Here's how the part is built. I have some questions about the finished solid (model axes, mm). Face numbers are marked on the shaded views. A direction names the side the tool comes from. Coordinates: 2 decimals unless noted, no trailing zeros. Write each loop counter-clockwise with the first axis right and the second up, starting at its lowest first coordinate (ties: lowest second). Pieces come first, ordered by that corner, then holes. Notation, with made-up numbers: M 26.25,-9 L 62.25,-9 A26 ccw 62.25,28 Z; hole C 87,-39.75 d11. An arc over 180 degrees is marked long. Use one line per item in the form item = value. Start each with the question number.
1. I want a section at A-A, the plane x = -18.5. List the corners of the cut face in (y, z) for me.
2. I want a section at D-D, the plane z = 45.5. List the corners of the cut face in (x, y) for me.
3. I want a section at C-C, the plane z = 55. List the corners of the cut face in (x, y) for me, plus the area to 3 significant figures.
4. Thinking about a two-plate mould opening in Z: for the marked faces 5, 6 and 7, which applies, released by +Z, released by -Z, zero draft, split by the parting line, or undercut?
5. I want a section at B-B, the plane z = 12. List the corners of the cut face in (x, y) for me.
6. I'm going to push flat-ended pins straight in: pin 1 Ø4.5 at (x, z) = (30.5, 56.5) entering from -Y; pin 2 Ø5 at (x, y) = (30, -9.5) entering from +Z; pin 3 Ø1 at (x, y) = (21, -24) entering from +Z. Where does each tip first touch, or does it pass through?
7. On a 3-axis mill with a long thin cutter (end or side, diameter ignored), from which of +Z, -Z, +X, -X, +Y, -Y can I reach the whole of each face in a straight line? I mean the marked faces 1, 2, 3 and 4. Say none if no direction works.
8. Please list where these lines run through material, in increasing order: line 1 along Z through (x, y) = (-32, -13); line 2 along X through (y, z) = (-7, 3); line 3 along X through (y, z) = (-4, 9). Write a range as [from, to].
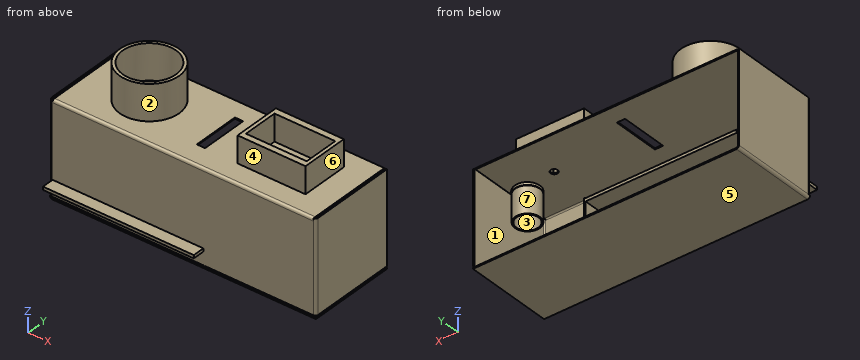
from build123d import *

# Parameters (mm, degrees)
SKETCH1_W                    = 150
SKETCH1_H                    = 50
BASE_FLANGE1_DEPTH           = 0.7366
EDGE_FLANGE2_STRIP_W         = 4.4196
EDGE_FLANGE2_STRIP_H         = 0.7366
EDGE_FLANGE2_STRIP_CUT_DEPTH = 50
EDGE_FLANGE2_DEPTH           = 50
EDGE_FLANGE3_STRIP_W         = 4.4196
EDGE_FLANGE3_STRIP_H         = 0.7366
EDGE_FLANGE3_STRIP_CUT_DEPTH = 51.7366
EDGE_FLANGE3_DEPTH           = 51.7366
EDGE_FLANGE5_STRIP_W         = 4.4196
EDGE_FLANGE5_STRIP_H         = 0.7366
EDGE_FLANGE5_STRIP_CUT_DEPTH = 51.7366
EDGE_FLANGE5_DEPTH           = 51.7366
EDGE_FLANGE6_STRIP_W         = 4.4196
EDGE_FLANGE6_STRIP_H         = 0.7366
EDGE_FLANGE6_STRIP_CUT_DEPTH = 147.0536
EDGE_FLANGE6_DEPTH           = 147.0536
SKETCH38_W                   = 4.66509895
SKETCH38_H                   = 26.811141958
CUT_EXTRUDE1_DEPTH           = 2
SKETCH40_R                   = 16.736303479
SKETCH40_R_2                 = 14.955594907
BOSS_EXTRUDE4_DEPTH          = 20
SKETCH42_W                   = 0.865074657
SKETCH42_H                   = 50
BOSS_EXTRUDE5_DEPTH          = 10
SKETCH57_W                   = 1.770321067
SKETCH57_H                   = 56.722896859
BOSS_EXTRUDE7_DEPTH          = 85
SKETCH60_W                   = 38.271407539
SKETCH60_H                   = 26.924897386
SKETCH60_W_2                 = 34.235775553
SKETCH60_H_2                 = 20.047107357
BOSS_EXTRUDE8_DEPTH          = 15
SKETCH61_R                   = 2.019782533
CUT_EXTRUDE3_DEPTH           = 2
SKETCH62_R                   = 1.571954748
BOSS_EXTRUDE9_DEPTH          = 3
SKETCH63_R                   = 7.10603058
BOSS_EXTRUDE10_DEPTH         = 1.5
SKETCH64_R                   = 6.980489156
SKETCH64_R_2                 = 6.226740222
BOSS_EXTRUDE11_DEPTH         = 15


# Sheet-metal steps are written as plain solids
with BuildPart() as part:
    # Sketch1 → Base-Flange1 (new body)
    with BuildSketch(Plane.XY):
        Rectangle(SKETCH1_W, SKETCH1_H)
    extrude(amount=-BASE_FLANGE1_DEPTH)

    # Edge-Flange2 strip (across the edge) → Edge-Flange2 strip cut (cut)
    with BuildSketch(Plane(origin=(-75, 25, 0), x_dir=(1, 0, 0), z_dir=(0, -1, 0))):
        with Locations((-0.7366, -0.3683)):
            Rectangle(EDGE_FLANGE2_STRIP_W, EDGE_FLANGE2_STRIP_H)
    extrude(amount=EDGE_FLANGE2_STRIP_CUT_DEPTH, mode=Mode.SUBTRACT)

    # Edge-Flange2 section (across the edge) → Edge-Flange2 (add)
    with BuildSketch(Plane(origin=(-75, 25, 0), x_dir=(1, 0, 0), z_dir=(0, -1, 0))):
        with BuildLine():
            Line((0, 0.7366), (0, 52.4732))
            Line((0, 52.4732), (0.7366, 52.4732))
            Line((0.7366, 52.4732), (0.7366, 0.7366))
            ThreePointArc((0.7366, 0.7366), (0.952345145, 0.215745145), (1.4732, 0))
            Line((1.4732, 0), (1.4732, -0.7366))
            ThreePointArc((1.4732, -0.7366), (0.43149029, -0.30510971), (0, 0.7366))
        make_face()
    extrude(amount=EDGE_FLANGE2_DEPTH)

    # Edge-Flange3 strip (across the edge) → Edge-Flange3 strip cut (cut)
    with BuildSketch(Plane(origin=(-74.2634, -25, 52.4732), x_dir=(0, 1, 0), z_dir=(0, 0, -1))):
        with Locations((-0.7366, -0.3683)):
            Rectangle(EDGE_FLANGE3_STRIP_W, EDGE_FLANGE3_STRIP_H)
    extrude(amount=EDGE_FLANGE3_STRIP_CUT_DEPTH, mode=Mode.SUBTRACT)

    # Edge-Flange3 section (across the edge) → Edge-Flange3 (add)
    with BuildSketch(Plane(origin=(-74.2634, -25, 52.4732), x_dir=(0, 1, 0), z_dir=(0, 0, -1))):
        with BuildLine():
            Line((0, 0.7366), (0, 149.2634))
            Line((0, 149.2634), (0.7366, 149.2634))
            Line((0.7366, 149.2634), (0.7366, 0.7366))
            ThreePointArc((0.7366, 0.7366), (0.952345145, 0.215745145), (1.4732, 0))
            Line((1.4732, 0), (1.4732, -0.7366))
            ThreePointArc((1.4732, -0.7366), (0.43149029, -0.30510971), (0, 0.7366))
        make_face()
    extrude(amount=EDGE_FLANGE3_DEPTH)

    # Edge-Flange5 strip (across the edge) → Edge-Flange5 strip cut (cut)
    with BuildSketch(Plane(origin=(75, -24.2634, 52.4732), x_dir=(-1, 0, 0), z_dir=(0, 0, -1))):
        with Locations((-0.7366, -0.3683)):
            Rectangle(EDGE_FLANGE5_STRIP_W, EDGE_FLANGE5_STRIP_H)
    extrude(amount=EDGE_FLANGE5_STRIP_CUT_DEPTH, mode=Mode.SUBTRACT)

    # Edge-Flange5 section (across the edge) → Edge-Flange5 (add)
    with BuildSketch(Plane(origin=(75, -24.2634, 52.4732), x_dir=(-1, 0, 0), z_dir=(0, 0, -1))):
        with BuildLine():
            Line((0, 0.7366), (0, 49.2634))
            Line((0, 49.2634), (0.7366, 49.2634))
            Line((0.7366, 49.2634), (0.7366, 0.7366))
            ThreePointArc((0.7366, 0.7366), (0.952345145, 0.215745145), (1.4732, 0))
            Line((1.4732, 0), (1.4732, -0.7366))
            ThreePointArc((1.4732, -0.7366), (0.43149029, -0.30510971), (0, 0.7366))
        make_face()
    extrude(amount=EDGE_FLANGE5_DEPTH)

    # Edge-Flange6 strip (across the edge) → Edge-Flange6 strip cut (cut)
    with BuildSketch(Plane(origin=(-73.5268, -24.2634, 52.4732), x_dir=(0, 0, -1), z_dir=(1, 0, 0))):
        with Locations((-0.7366, -0.3683)):
            Rectangle(EDGE_FLANGE6_STRIP_W, EDGE_FLANGE6_STRIP_H)
    extrude(amount=EDGE_FLANGE6_STRIP_CUT_DEPTH, mode=Mode.SUBTRACT)

    # Edge-Flange6 section (across the edge) → Edge-Flange6 (add)
    with BuildSketch(Plane(origin=(-73.5268, -24.2634, 52.4732), x_dir=(0, 0, -1), z_dir=(1, 0, 0))):
        with BuildLine():
            Line((0, 0.7366), (0, 49.2634))
            Line((0, 49.2634), (0.7366, 49.2634))
            Line((0.7366, 49.2634), (0.7366, 0.7366))
            ThreePointArc((0.7366, 0.7366), (0.952345145, 0.215745145), (1.4732, 0))
            Line((1.4732, 0), (1.4732, -0.7366))
            ThreePointArc((1.4732, -0.7366), (0.43149029, -0.30510971), (0, 0.7366))
        make_face()
    extrude(amount=EDGE_FLANGE6_DEPTH)

    # Sketch38 → Cut-Extrude1 (cut)
    with BuildSketch(Plane.XY.offset(52.4732)):
        with Locations((0, 1.125354672)):
            Rectangle(SKETCH38_W, SKETCH38_H)
    extrude(amount=-CUT_EXTRUDE1_DEPTH, mode=Mode.SUBTRACT)

    # Sketch40 → Boss-Extrude4 (add)
    with BuildSketch(Plane.XY.offset(52.4732)):
        with Locations((-40.204479975, 1.659887055)):
            Circle(SKETCH40_R)
        with Locations((-40.204479975, 1.659887055)):
            Circle(SKETCH40_R_2, mode=Mode.SUBTRACT)
    extrude(amount=BOSS_EXTRUDE4_DEPTH)

    # Sketch42 → Boss-Extrude5 (add)
    with BuildSketch(Plane.XY):
        with Locations((11.975597677, 0)):
            Rectangle(SKETCH42_W, SKETCH42_H)
    extrude(amount=BOSS_EXTRUDE5_DEPTH)

    # Sketch57 → Boss-Extrude7 (add)
    with BuildSketch(Plane.ZY.offset(-11.543060348)):
        with Locations((8.882085538, -3.36144843)):
            Rectangle(SKETCH57_W, SKETCH57_H)
    extrude(amount=BOSS_EXTRUDE7_DEPTH)

    # Sketch60 → Boss-Extrude8 (add)
    with BuildSketch(Plane.XY.offset(52.4732)):
        with Locations((40.051357612, 0.865314599)):
            Rectangle(SKETCH60_W, SKETCH60_H)
        with Locations((40.096607613, 0.750841138)):
            Rectangle(SKETCH60_W_2, SKETCH60_H_2, mode=Mode.SUBTRACT)
    extrude(amount=BOSS_EXTRUDE8_DEPTH)

    # Sketch61 → Cut-Extrude3 (cut)
    with BuildSketch(Plane(origin=(0, 0, 51.7366), x_dir=(-1, 0, 0), z_dir=(0, 0, -1))):
        with Locations((-47.658560575, 2.019782533)):
            Circle(SKETCH61_R)
    extrude(amount=-CUT_EXTRUDE3_DEPTH, mode=Mode.SUBTRACT)

    # Sketch62 → Boss-Extrude9 (add)
    with BuildSketch(Plane(origin=(0, 0, 51.7366), x_dir=(-1, 0, 0), z_dir=(0, 0, -1))):
        with Locations(Location((-63.948086172, 1.147200329, 0), (0, 0, 180))):
            Circle(SKETCH62_R)
    extrude(amount=BOSS_EXTRUDE9_DEPTH)

    # Sketch63 → Boss-Extrude10 (add)
    with BuildSketch(Plane(origin=(0, 0, 48.7366), x_dir=(-1, 0, 0), z_dir=(0, 0, -1))):
        with Locations((-63.631248371, 0.988840217)):
            Circle(SKETCH63_R)
    extrude(amount=BOSS_EXTRUDE10_DEPTH)

    # Sketch64 → Boss-Extrude11 (add)
    with BuildSketch(Plane(origin=(0, 0, 47.2366), x_dir=(-1, 0, 0), z_dir=(0, 0, -1))):
        with Locations(Location((-63.746933468, 0.733116553, 0), (0, 0, 181.202812621))):
            Circle(SKETCH64_R)
        with Locations((-63.746933468, 0.733116553)):
            Circle(SKETCH64_R_2, mode=Mode.SUBTRACT)
    extrude(amount=BOSS_EXTRUDE11_DEPTH)


solid = part.part
Answer list:
q1.outline = M -31.72,8 L -25,8 L -25,0.74 L -24.26,0.74 L -24.26,8 L 25,8 L 25,9.77 L -24.26,9.77 L -24.26,51 A0.74 cw -23.53,51.74 L 25,51.74 L 25,52.47 L -23.53,52.47 A1.47 ccw -25,51 L -25,9.77 L -31.72,9.77 Z; M -25,-0.74 L 25,-0.74 L 25,0 L -25,0 Z
q2.outline = M -75,-23.53 A1.47 ccw -73.53,-25 L 73.53,-25 A1.47 ccw 75,-23.53 L 75,25 L 74.26,25 L 74.26,-23.53 A0.74 cw 73.53,-24.26 L -73.53,-24.26 A0.74 cw -74.26,-23.53 L -74.26,25 L -75,25 Z; C 63.75,0.73 d13.96; hole C 63.75,0.73 d12.45
q3.outline = C -40.2,1.66 d33.47; M 20.92,-12.6 L 59.19,-12.6 L 59.19,14.33 L 20.92,14.33 Z; hole C -40.2,1.66 d29.91; hole M 22.98,-9.27 L 57.21,-9.27 L 57.21,10.77 L 22.98,10.77 Z
q3.area = 521 mm²
q4.face_5 = released by -Z
q4.face_6 = zero draft
q4.face_7 = undercut
q5.outline = M -75,-23.53 A1.47 ccw -73.53,-25 L 73.53,-25 A1.47 ccw 75,-23.53 L 75,25 L 74.26,25 L 74.26,-23.53 A0.74 cw 73.53,-24.26 L -73.53,-24.26 A0.74 cw -74.26,-23.53 L -74.26,25 L -75,25 Z
q6.pin_1 = -12.6
q6.pin_2 = 67.47
q6.pin_3 = 52.47
q7.face_1 = +Z, +Y
q7.face_2 = +Z
q7.face_3 = none
q7.face_4 = +Z, +X, -Y
q8.line_1 = [-0.74, 0], [8, 9.77], [51.74, 52.47]
q8.line_2 = [-75, -74.26], [11.54, 12.41], [74.26, 75]
q8.line_3 = [-75, -74.26], [-73.46, 12.41], [74.26, 75]
